```python
from build123d import *

# Parameters (mm, degrees)
CROQUIS1_R              = 217.5
SALIENTE_EXTRUIR1_DEPTH = 125
REDONDEO2_R             = 62.5
CORTAR_EXTRUIR4_DEPTH   = 115


with BuildPart() as part:
    # Croquis1 → Saliente-Extruir1 (new body)
    with BuildSketch(Plane.XY):
        with Locations((-1.153997035, 0)):
            Circle(CROQUIS1_R)
    extrude(amount=SALIENTE_EXTRUIR1_DEPTH)

    # Redondeo2
    redondeo2_edges = [part.edges().sort_by_distance(p)[0] for p in [
        (-218.653997035, 0, 0),
        (-218.653997035, 0, 125),
    ]]
    fillet(redondeo2_edges, radius=REDONDEO2_R - 0.0001)  # a hair under: the kernel refuses the full size

    # Croquis6 → Cortar-Extruir4 (cut)
    with BuildSketch(Plane.XY.offset(125)):
        with BuildLine():
            ThreePointArc((148.115736426, 5), (104.793299826, 104.793299826), (5, 148.115736426))
            Line((5, 148.115736426), (5, 133.106229009))
            ThreePointArc((5, 133.106229009), (94.186698108, 94.186698108), (133.106229009, 5))
            Line((133.106229009, 5), (148.115736426, 5))
        make_face()
        with BuildLine():
            ThreePointArc((5, -148.115736426), (104.793299826, -104.793299826), (148.115736426, -5))
            Line((148.115736426, -5), (133.106229009, -5))
            ThreePointArc((133.106229009, -5), (94.186698108, -94.186698108), (5, -133.106229009))
            Line((5, -133.106229009), (5, -148.115736426))
        make_face()
        with BuildLine():
            Line((-133.106229009, -5), (-148.115736426, -5))
            ThreePointArc((-148.115736426, -5), (-104.793299826, -104.793299826), (-5, -148.115736426))
            Line((-5, -148.115736426), (-5, -133.106229009))
            ThreePointArc((-5, -133.106229009), (-94.186698108, -94.186698108), (-133.106229009, -5))
        make_face()
        with BuildLine():
            Line((-5, 133.106229009), (-5, 148.115736426))
            ThreePointArc((-5, 148.115736426), (-104.793299826, 104.793299826), (-148.115736426, 5))
            Line((-148.115736426, 5), (-133.106229009, 5))
            ThreePointArc((-133.106229009, 5), (-94.186698108, 94.186698108), (-5, 133.106229009))
        make_face()
        with BuildLine():
            Line((-5, 113.089628024), (-5, 128.102564933))
            ThreePointArc((-5, 128.102564933), (-90.651164202, 90.651164202), (-128.102564933, 5))
            Line((-128.102564933, 5), (-113.089628024, 5))
            ThreePointArc((-113.089628024, 5), (-80.044562485, 80.044562485), (-5, 113.089628024))
        make_face()
        with BuildLine():
            Line((-113.089628024, -5), (-128.102564933, -5))
            ThreePointArc((-128.102564933, -5), (-90.651164202, -90.651164202), (-5, -128.102564933))
            Line((-5, -128.102564933), (-5, -113.089628024))
            ThreePointArc((-5, -113.089628024), (-80.044562485, -80.044562485), (-113.089628024, -5))
        make_face()
        with BuildLine():
            Line((-5, 93.065889198), (-5, 108.08451743))
            ThreePointArc((-5, 108.08451743), (-76.509028579, 76.509028579), (-108.08451743, 5))
            Line((-108.08451743, 5), (-93.065889198, 5))
            ThreePointArc((-93.065889198, 5), (-65.902426861, 65.902426861), (-5, 93.065889198))
        make_face()
        with BuildLine():
            Line((-93.065889198, -5), (-108.08451743, -5))
            ThreePointArc((-108.08451743, -5), (-76.509028579, -76.509028579), (-5, -108.08451743))
            Line((-5, -108.08451743), (-5, -93.065889198))
            ThreePointArc((-5, -93.065889198), (-65.902426861, -65.902426861), (-93.065889198, -5))
        make_face()
        with BuildLine():
            Line((-58.540309792, -5), (-73.58377108, -5))
            ThreePointArc((-73.58377108, -5), (-52.151564532, -52.151564532), (-5, -73.58377108))
            Line((-5, -73.58377108), (-5, -58.540309792))
            ThreePointArc((-5, -58.540309792), (-41.544962815, -41.544962815), (-58.540309792, -5))
        make_face()
        with BuildLine():
            Line((-5, 58.540309792), (-5, 73.58377108))
            ThreePointArc((-5, 73.58377108), (-52.151564532, 52.151564532), (-73.58377108, 5))
            Line((-73.58377108, 5), (-58.540309792, 5))
            ThreePointArc((-58.540309792, 5), (-41.544962815, 41.544962815), (-5, 58.540309792))
        make_face()
        with BuildLine():
            Line((-5, 78.594566383), (-5, 88.058268628))
            ThreePointArc((-5, 88.058268628), (-62.366892955, 62.366892955), (-88.058268628, 5))
            Line((-88.058268628, 5), (-78.594566383, 5))
            ThreePointArc((-78.594566383, 5), (-55.687098438, 55.687098438), (-5, 78.594566383))
        make_face()
        with BuildLine():
            Line((-78.594566383, -5), (-88.058268628, -5))
            ThreePointArc((-88.058268628, -5), (-62.366892955, -62.366892955), (-5, -88.058268628))
            Line((-5, -88.058268628), (-5, -78.594566383))
            ThreePointArc((-5, -78.594566383), (-55.687098438, -55.687098438), (-78.594566383, -5))
        make_face()
        with BuildLine():
            Line((-38.429544313, -5), (-53.520401455, -5))
            ThreePointArc((-53.520401455, -5), (-38.009428909, -38.009428909), (-5, -53.520401455))
            Line((-5, -53.520401455), (-5, -38.429544313))
            ThreePointArc((-5, -38.429544313), (-27.402827191, -27.402827191), (-38.429544313, -5))
        make_face()
        with BuildLine():
            Line((-5, 38.429544313), (-5, 53.520401455))
            ThreePointArc((-5, 53.520401455), (-38.009428909, 38.009428909), (-53.520401455, 5))
            Line((-53.520401455, 5), (-38.429544313, 5))
            ThreePointArc((-38.429544313, 5), (-27.402827191, 27.402827191), (-5, 38.429544313))
        make_face()
        with BuildLine():
            ThreePointArc((5, -53.520401455), (38.009428909, -38.009428909), (53.520401455, -5))
            Line((53.520401455, -5), (38.429544313, -5))
            ThreePointArc((38.429544313, -5), (27.402827191, -27.402827191), (5, -38.429544313))
            Line((5, -38.429544313), (5, -53.520401455))
        make_face()
        with BuildLine():
            ThreePointArc((53.520401455, 5), (38.009428909, 38.009428909), (5, 53.520401455))
            Line((5, 53.520401455), (5, 38.429544313))
            ThreePointArc((5, 38.429544313), (27.402827191, 27.402827191), (38.429544313, 5))
            Line((38.429544313, 5), (53.520401455, 5))
        make_face()
        with BuildLine():
            ThreePointArc((73.58377108, 5), (52.151564532, 52.151564532), (5, 73.58377108))
            Line((5, 73.58377108), (5, 58.540309792))
            ThreePointArc((5, 58.540309792), (41.544962815, 41.544962815), (58.540309792, 5))
            Line((58.540309792, 5), (73.58377108, 5))
        make_face()
        with BuildLine():
            ThreePointArc((88.058268628, 5), (62.366892955, 62.366892955), (5, 88.058268628))
            Line((5, 88.058268628), (5, 78.594566383))
            ThreePointArc((5, 78.594566383), (55.687098438, 55.687098438), (78.594566383, 5))
            Line((78.594566383, 5), (88.058268628, 5))
        make_face()
        with BuildLine():
            ThreePointArc((108.08451743, 5), (76.509028579, 76.509028579), (5, 108.08451743))
            Line((5, 108.08451743), (5, 93.065889198))
            ThreePointArc((5, 93.065889198), (65.902426861, 65.902426861), (93.065889198, 5))
            Line((93.065889198, 5), (108.08451743, 5))
        make_face()
        with BuildLine():
            ThreePointArc((128.102564933, 5), (90.651164202, 90.651164202), (5, 128.102564933))
            Line((5, 128.102564933), (5, 113.089628024))
            ThreePointArc((5, 113.089628024), (80.044562485, 80.044562485), (113.089628024, 5))
            Line((113.089628024, 5), (128.102564933, 5))
        make_face()
        with BuildLine():
            ThreePointArc((5, -128.102564933), (90.651164202, -90.651164202), (128.102564933, -5))
            Line((128.102564933, -5), (113.089628024, -5))
            ThreePointArc((113.089628024, -5), (80.044562485, -80.044562485), (5, -113.089628024))
            Line((5, -113.089628024), (5, -128.102564933))
        make_face()
        with BuildLine():
            ThreePointArc((5, -108.08451743), (76.509028579, -76.509028579), (108.08451743, -5))
            Line((108.08451743, -5), (93.065889198, -5))
            ThreePointArc((93.065889198, -5), (65.902426861, -65.902426861), (5, -93.065889198))
            Line((5, -93.065889198), (5, -108.08451743))
        make_face()
        with BuildLine():
            ThreePointArc((5, -88.058268628), (62.366892955, -62.366892955), (88.058268628, -5))
            Line((88.058268628, -5), (78.594566383, -5))
            ThreePointArc((78.594566383, -5), (55.687098438, -55.687098438), (5, -78.594566383))
            Line((5, -78.594566383), (5, -88.058268628))
        make_face()
        with BuildLine():
            ThreePointArc((5, -73.58377108), (52.151564532, -52.151564532), (73.58377108, -5))
            Line((73.58377108, -5), (58.540309792, -5))
            ThreePointArc((58.540309792, -5), (41.544962815, -41.544962815), (5, -58.540309792))
            Line((5, -58.540309792), (5, -73.58377108))
        make_face()
    extrude(amount=-CORTAR_EXTRUIR4_DEPTH, mode=Mode.SUBTRACT)


solid = part.part
```
Verification items for the finished model (mm, model axes). Give positions to 0.01 mm unless a question says otherwise; leave off trailing zeros. Put each result on its own line as item: value.
Q1. Depth check by flat-ended pin: P1, Ø1, axis at x = -31, z = 109.5, coming from the +Y side; P2, Ø12, axis at y = 103, z = 72.5, coming from the +X side; P3, Ø5, axis at y = 32.5, z = 48, coming from the -X side. Enter the tip coordinate at first touch or a pass-through.
Result:
P1: y = 194.49
P2: x = 192.78
P3: x = -215.16
Q2. Scan lines: probe 1 along X at (y, z) = (-119, 25); probe 2 along Z at (x, y) = (146.5, 10.5); probe 3 along Z at (x, y) = (114, 106). Record each from-to range of solid material in increasing order. Write a range as from..to.
Result:
probe 1: -168.08..-88.33, -59.84..-47.69, -5..5, 47.69..59.84, 88.33..165.77
probe 2: 0..10
probe 3: 0.02..124.98
Q3. Section check A-A on z = 109. Count the separate pieces of the cut face and the enclosed holes in it, and give its area (3 significant figures).
Result:
separate pieces: 1
enclosed holes: 24
area: 75,300 mm2
